Could you check a few things on this model? Use its own coordinates, in mm. A direction names the side the tool comes from. Give positions to 0.01 mm unless a question says otherwise; leave off trailing zeros. Write each loop counter-clockwise with the first axis right and the second up, starting at its lowest first coordinate (ties: lowest second). Pieces come first, ordered by that corner, then holes. Notation, with made-up numbers: M 79.5,43.25 L 92.5,43.25 A22 ccw 92.5,68.25 Z; hole C 27.25,46.5 d11. An arc over 180 degrees is marked long. One line per item, written item: value.
```python
from build123d import *

# Parameters (mm, degrees)
F1_DEPTH = 9.398
F3_DEPTH = 15.24


with BuildPart() as f1:
    # F0 (on Top) → F1 (new body)
    with BuildSketch(Plane.XY):
        Polygon((0, 38.1), (0, 0), (1.5875, 0), (1.5875, 13.8176), (15.9385, 13.8176), (15.9385, 0), (17.526, 0), (17.526, 38.1), align=None)
    extrude(amount=F1_DEPTH)

    # F2 (on face) → F3 (cut)
    with BuildSketch(Plane(origin=(0, 38.1, 0), x_dir=(-1, 0, 0), z_dir=(0, 1, 0))):
        with BuildLine():
            Line((-13.0094570703, 9.398), (-13.0094570703, 7.2687586724))
            ThreePointArc((-13.0094570703, 7.2687586724), (-8.647429717, 2.7979053307), (-4.5347851701, 7.4991782504))
            Line((-4.5347851701, 7.4991782504), (-4.5347851701, 9.398))
            Line((-4.5347851701, 9.398), (-13.0094570703, 9.398))
        make_face()
    extrude(amount=-F3_DEPTH, mode=Mode.SUBTRACT)


solid = f1.part
```
1) If we section it at C-C, the plane y = 34: Write out the boundary of the cut face in (x, z).
Outcome:
outline: M 0,0 L 17.53,0 L 17.53,9.4 L 13.01,9.4 L 13.01,7.27 A4.25 cw long 4.53,7.5 L 4.53,9.4 L 0,9.4 Z
2) If we section it at B-B, the plane z = 8.75: Write out the boundary of the cut face in (x, y).
Outcome:
outline: M 0,0 L 1.59,0 L 1.59,13.82 L 15.94,13.82 L 15.94,0 L 17.53,0 L 17.53,38.1 L 13.01,38.1 L 13.01,22.86 L 4.53,22.86 L 4.53,38.1 L 0,38.1 Z
3) Please list where these lines run through material, in increasing order: L1, parallel to X at y = 34, z = 7; L2, parallel to X at y = 10, z = 6.25; L3, parallel to Y at x = 8.5, z = 8.25. Write a range as from..to.
Outcome:
L1: x = 0..4.51, 13.01..17.53
L2: x = 0..1.59, 15.94..17.53
L3: y = 13.82..22.86
4) If we section it at A-A, the plane y = 3: Write out the boundary of the cut face in (x, z), then the cut area to 3 significant figures.
Outcome:
outline: M 0,0 L 1.59,0 L 1.59,9.4 L 0,9.4 Z; M 15.94,0 L 17.53,0 L 17.53,9.4 L 15.94,9.4 Z
area: 29.8 mm^2
5) If we section it at D-D, the plane x = 14.5: Write out the boundary of the cut face in (y, z), then the cut area to 3 significant figures.
Outcome:
outline: M 13.82,0 L 38.1,0 L 38.1,9.4 L 13.82,9.4 Z
area: 228 mm^2
6) On a 3-axis mill with a long thin cutter (end or side, diameter ignored), from which of +Z, -Z, +X, -X, +Y, -Y can I reach the whole of each face in a straight line? I mean faces 1 (the face through (9, 13.818, 5)), 2 (the face through (9, 24, 0)), 3 (the face through (4.535, 31, 8)). Say none if no direction works.
Outcome:
face 1: +Z, -Z, -Y
face 2: -Z, +X, -X, +Y, -Y
face 3: +Z, +Y
7) I'm going to push flat-ended pins straight in: pin 1 (3.5 mm diameter, centred on x = 9, z = 6.5, fed in from +Y); pin 2 (3 mm diameter, centred on x = 12, z = 8.5, fed in from -Y). Where does each tip first touch, or does it pass through?
Outcome:
pin 1: stops at y = 22.86
pin 2: stops at y = 13.82
